Geometry check sheet. Reference: the model listing, model coordinates, mm. Coordinates: 2 decimals unless noted, no trailing zeros. Write each loop counter-clockwise with the first axis right and the second up, starting at its lowest first coordinate (ties: lowest second). Pieces come first, ordered by that corner, then holes.
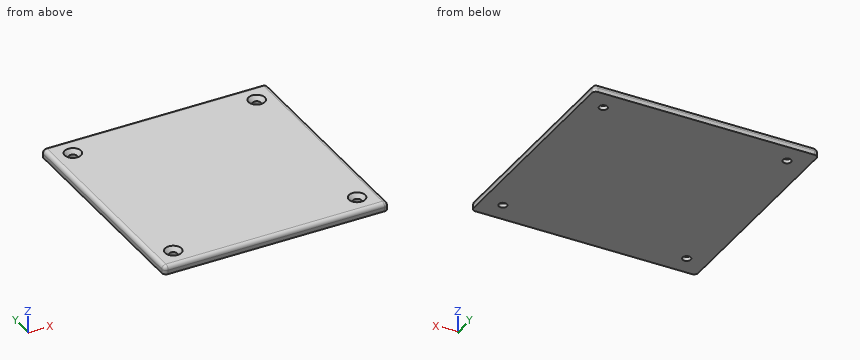
Autodesk Inventor part; units mm, degrees
ref_plane "YZ Plane" through (0, 0, 0) normal (1, 0, 0) x (0, 1, 0)
ref_plane "XZ Plane" through (0, 0, 0) normal (0, 1, 0) x (-1, 0, 0)
ref_plane "XY Plane" through (0, 0, 0) normal (0, 0, 1) x (1, 0, 0)
sketch "Sketch2" plane through (0, 0, 0) normal (0, 0, 1) x (1, 0, 0)
  line L0 (-55, -55) -> (55, -55)
  line L1 (55, -55) -> (55, 55)
  line L2 (55, 55) -> (-55, 55)
  line L3 (-55, 55) -> (-55, -55)
  line L4 (-55, -55) -> (55, 55) construction
  line L5 (55, -55) -> (-55, 55) construction
  point P0 (0, 0)
  dimension "Lid_Width" = 110
  dimension "Lid_Length" = 110
extrude "Extrusion1" add sketch "Sketch2" along normal blind 4
fillet "Fillet1" radius 2 8 edges at (-55, -55, 2) (-55, 55, 2) (55, 55, 2) (55, -55, 2) (55, 0, 4) (0, 55, 4) (-55, 0, 4) (0, -55, 4)
sketch "Sketch6" plane through (0, 0, 4) normal (0, 0, 1) x (1, 0, 0)
  circle A0 centre (-45, 45) radius 2
  line L0 (53, 55) -> (-53, 55)
  line L1 (-55, 53) -> (-55, -53)
  line L2 (0, 0) -> (0, 55) construction
  line L3 (0, 0) -> (-55, 0) construction
  circle A1 centre (45, 45) radius 2
  circle A2 centre (-45, -45) radius 2
  circle A3 centre (45, -45) radius 2
  dimension "d26" = 4
  dimension "d27" = 10
  dimension "d28" = 10
extrude "Extrusion4" cut sketch "Sketch6" against normal blind 4
chamfer "Chamfer2" distance 2 angle 45 4 edges at (-47, 45, 4) (43, 45, 4) (43, -45, 4) (-47, -45, 4)
equation "\"Lid_Width\" = PCB_Width + 2 * Offset"
equation "\"Lid_Length\" = PCB_Length + 2 * Offset"
equation "\"d2\" = 2 * Wall_Thickness"
equation "\"d4\" = Wall_Thickness"
equation "\"d29\" = 2 * Wall_Thickness"
equation "\"d31\" = Wall_Thickness"
equation "\"Offset\" = 15"
equation "\"Wall_Thickness\" = 2"
properties part number "Lid"
1. Thickness scan on line 1 along Y through (x, z) = (45, 0.5); line 2 along Y through (x, z) = (43, 2.7); line 3 along X through (y, z) = (12, 2.2). Record the ranges inside material, lowest first.
Computed values:
line 1: y = -55 to -47, -43 to 43, 47 to 55
line 2: y = -54.87 to -46.81, -43.19 to 43.19, 46.81 to 54.87
line 3: x = -54.99 to 54.99
2. Gauge pin test, flat end, axial feed: pin 1 Ø2.5 at (x, y) = (45, -45) entering from -Z. Record the tip position at first contact, or that the pin passes through.
Computed values:
pin 1: passes through
3. Sectioned sample at A-A, the plane x = -45. Record the boundary of the cut face in (y, z), and give its area (3 significant figures).
Computed values:
outline: (-55, 0) - (-47, 0) - (-47, 2) - (-49, 4) - (-53, 4) arc R2 ccw to (-55, 2) - close; (-43, 0) - (43, 0) - (43, 2) - (41, 4) - (-41, 4) - (-43, 2) - close; (47, 0) - (55, 0) - (55, 2) arc R2 ccw to (53, 4) - (49, 4) - (47, 2) - close
area: 398 mm2
